The listing builds one solid part. Answer for the finished solid, in the listing's coordinates (mm). A direction names the side the tool comes from. Coordinates: 2 decimals unless noted, no trailing zeros. Write each loop counter-clockwise with the first axis right and the second up, starting at its lowest first coordinate (ties: lowest second). Pieces come first, ordered by that corner, then holes. Notation, with made-up numbers: M 44,75 L 61,75 A20 cw 61,105 Z; hole C 59,-28.75 d4. An arc over 180 degrees is marked long. Put each result on its own line as item: value. Start each with the question number.
```python
from build123d import *

# Parameters (mm, degrees)
F0_W     = 77.10462
F0_H     = 35.696581
F1_DEPTH = 25.4
F4_DEPTH = 109.789906


with BuildPart() as f1:
    # F0 (on Front) → F1 (new body)
    with BuildSketch(Plane.XZ):
        with Locations((-2.284579, 38.12395)):
            Rectangle(F0_W, F0_H)
    extrude(amount=F1_DEPTH)

    # F3 (on face) → F4 (join)
    with BuildSketch(Plane.XZ):
        Polygon((-146.92077, -19.15716), (-45.091689, -19.15716), (-45.091689, -11.375816), (-38.160954, -11.375816), (-38.160954, 75.124502), (-146.92077, 75.124502), align=None)
    extrude(amount=F4_DEPTH)


solid = f1.part
```
1) A cutting plane is placed at D-D on y = -56.5. Write down the section's boundary in (x, z), then the cut area to 3 significant figures.
2) A cutting plane is placed at C-C on x = 10.5. Write down the section's boundary in (y, z), then the cut area to 3 significant figures.
3) A cutting plane is placed at B-B on z = 45. Write down the section's boundary in (x, y), then the cut area to 3 significant figures.
4) Determine the mould class of faces 1 (the face through (-146.921, -54, 29)), 2 (the face through (-45.092, -54, -15)), 3 (the face through (-1, -13, 20.276)) for opening direction X: +X half, -X half, draft (parallel to the pull), parting line (faces both ways), or undercut.
5) A cutting plane is placed at A-A on y = -13. Write down the section's boundary in (x, z).
6) For faces 4 (the face through (-42, -54, -11.376)), 5 (the face through (-1, -13, 55.972)), 6 (the face through (-1, -25.4, 38)), determine the directions among +Z, -Z, +X, -X, +Y, -Y from which every point of the face is accessible in a straight line to the end or side of a thin tool.
7) Given pin 1 Ø2.5 at (y, z) = (-59, -16) entering from +X; pin 2 Ø12.5 at (x, y) = (-3.5, -9) entering from +Z; pin 3 Ø3.5 at (x, y) = (-42.5, -33.5) entering from -Z, each flat-ended and moving along its own axis, determine where each tip first touches the part or whether it passes through.
8) Straight lines are drawn through the part: probe 1 along X at (y, z) = (-36, 71); probe 2 along Y at (x, z) = (9.5, 55). For each, find the intervals that lie inside material, in ascending order.
Answers follow:
1. outline: M -146.92,-19.16 L -45.09,-19.16 L -45.09,-11.38 L -38.16,-11.38 L -38.16,75.12 L -146.92,75.12 Z
1. area: 10,200 mm²
2. outline: M -25.4,20.28 L 0,20.28 L 0,55.97 L -25.4,55.97 Z
2. area: 907 mm²
3. outline: M -146.92,-109.79 L -38.16,-109.79 L -38.16,-25.4 L 36.27,-25.4 L 36.27,0 L -146.92,0 Z
3. area: 13,800 mm²
4. face 1: -X half
4. face 2: +X half
4. face 3: draft
5. outline: M -146.92,-19.16 L -45.09,-19.16 L -45.09,-11.38 L -38.16,-11.38 L -38.16,20.28 L 36.27,20.28 L 36.27,55.97 L -38.16,55.97 L -38.16,75.12 L -146.92,75.12 Z
6. face 4: -Z, +X, +Y, -Y
6. face 5: +Z, +X, +Y, -Y
6. face 6: +Z, -Z, +X, -Y
7. pin 1: stops at x = -45.09
7. pin 2: stops at z = 55.97
7. pin 3: stops at z = -11.38
8. probe 1: x = -146.92 to -38.16
8. probe 2: y = -25.4 to 0
